Autodesk Inventor part; units mm, degrees
ref_plane "Start plane" through (0, 0, 0) normal (0, 0, 1) x (1, 0, 0)
ref_plane "End plane" through (0, 0, 900) normal (0, 0, 1) x (1, 0, 0)
ref_plane "YZ Plane" through (0, 0, 0) normal (1, 0, 0) x (0, 1, 0)
ref_plane "Start plane" through (0, 0, 0) normal (0, 0, 1) x (1, 0, 0)
ref_plane "End plane" through (0, 0, 900) normal (0, 0, 1) x (1, 0, 0)
sketch "Sketch" plane through (0, 0, 0) normal (0, 0, 1) x (1, 0, 0)
  line L0 (0.8698, -38.5) -> (-0.8698, -38.5)
  line L1 (2.2911, -16.445) -> (1.8696, -37.52)
  line L2 (13.04, -12.3892) -> (6.2103, -12.5258)
  line L3 (15, -8.5) -> (15, -10.3896)
  line L4 (-15, -10.3896) -> (-15, -8.5)
  line L5 (-6.2103, -12.5258) -> (-13.04, -12.3892)
  line L6 (-1.8696, -37.52) -> (-2.2911, -16.445)
  line L7 (-2.3679, -12.6026) -> (2.3679, -12.6026) construction
  line L8 (0, -46.445) -> (0, 7.7408) construction
  arc A0 (-2.2911, -16.445) -> (-6.2103, -12.5258) centre (-6.2903, -16.525) ccw
  arc A1 (6.2103, -12.5258) -> (2.2911, -16.445) centre (6.2903, -16.525) ccw
  arc A2 (-15, -10.3896) -> (-13.04, -12.3892) centre (-13, -10.3896) ccw
  arc A3 (13.04, -12.3892) -> (15, -10.3896) centre (13, -10.3896) ccw
  arc A4 (-1.8696, -37.52) -> (-0.8698, -38.5) centre (-0.8698, -37.5) ccw
  arc A5 (0.8698, -38.5) -> (1.8696, -37.52) centre (0.8698, -37.5) ccw
  line L9 (-21.5716, 0) -> (21.5716, 0) construction
  line L10 (-15, -8.5) -> (15, -8.5)
  point P0 (1.85, -38.5)
  point P1 (-1.85, -38.5)
  point P2 (15, -12.35)
  point P3 (-15, -12.35)
  point P4 (0, 0)
  point P5 (0, -12.6026)
  dimension "d9" = 3.85
  dimension "d11" = 3.85
  dimension "d23" = 3.7
  dimension "d26" = 1.146
  dimension "d27" = 1.146
  dimension "d28" = 4
  dimension "d29" = 2
  dimension "d30" = 1
  dimension "d31" = 30
  dimension "d32" = 1.146
  dimension "d33" = 30
  dimension "d34" = 8.5
extrude "Body" add sketch "Sketch" along normal up to surface (900 mm away) from surface at 0
sketch "Sketch3" plane through (0, 0, 0) normal (0, 0, 1) x (1, 0, 0)
  line L0 (0, 0) -> (10, 0)
ref_plane "Work Plane6" through (0, 0, 0) normal (0, -1, 0) x (1, 0, 0)
sketch "Sketch4" plane through (0, 0, 0) normal (0, -1, 0) x (1, 0, 0)
  line L0 (-2, 0) -> (12, 0)
  line L1 (-2, 900) -> (12, 900)
  dimension "d38" = 900
equation "\"d26\" = d27"
equation "\"d27\" = d32"
equation "\"d28\" = R"
equation "\"d29\" = R1"
equation "\"d30\" = R2"
equation "\"d32\" = msp_ang"
equation "\"d33\" = b"
equation "\"d34\" = ex"
equation "\"d13\" = G_L"
equation "\"b\" = 30"
equation "\"ParH\" = 30"
equation "\"R\" = 4"
equation "\"ParT\" = 4"
equation "\"R1\" = 2"
equation "\"R2\" = 1"
equation "\"G_L\" = d38"
equation "\"msp_x1\" = 0"
equation "\"msp_x2\" = 0"
equation "\"msp_x\" = 0"
equation "\"msp_ang\" = 1.14576deg"
equation "\"ex\" = 8.5"
equation "\"G_OFFSET_START\" = 0"
equation "\"G_OFFSET_END\" = 0"
properties part number "DIN 1024 - T30-900" material "Steel, Mild"
Model file for the job. Use its own axes, mm. Coordinates: 2 decimals unless noted, no trailing zeros. Loops run counter-clockwise (first coordinate to the right, second up) from the corner with the lowest first, then second, coordinate; pieces in that order, holes last. Notation, with made-up numbers: (26.5, 44) - (77.5, 44) arc R17 ccw to (77.5, 72) - close; hole circle Ø9 at (60, 43.25). An arc over 180 degrees is marked (long way). Write item = value, one per line. Start each with the question number.
Item 1: Saw through at A-A, the plane z = 225. List the corners of the cut face in (x, y) (3 decimals).
Item 2: Drop flat-ended pins along their axis: pin 1 Ø2 at (x, z) = (11, 616) entering from -Y; pin 2 Ø4 at (y, z) = (-25, 272.5) entering from +X; pin 3 Ø10 at (y, z) = (-22, 299.5) entering from -X. Give the stop position or say it passes through.
Item 3: Saw through at B-B, the plane y = -29. List the corners of the cut face in (x, z).
Item 4: Wall check: probe 1 along X at (y, z) = (-29.75, 293.5) (3 decimals); probe 2 along Y at (x, z) = (-10.25, 814) (3 decimals); probe 3 along X at (y, z) = (-22, 652.5). Give the ranges that are in metal, low to high. Write a range as [from, to].
Answers:
q1.outline = (-15, -10.39) arc R2 ccw to (-13.04, -12.389) - (-6.21, -12.526) arc R4 cw to (-2.291, -16.445) - (-1.87, -37.52) arc R1 ccw to (-0.87, -38.5) - (0.87, -38.5) arc R1 ccw to (1.87, -37.52) - (2.291, -16.445) arc R4 cw to (6.21, -12.526) - (13.04, -12.389) arc R2 ccw to (15, -10.39) - (15, -8.5) - (-15, -8.5) - close
q2.pin_1 = -12.45
q2.pin_2 = 2.16
q2.pin_3 = -2.28
q3.outline = (-2.04, 0) - (2.04, 0) - (2.04, 900) - (-2.04, 900) - close
q4.probe_1 = [-2.025, 2.025]
q4.probe_2 = [-12.445, -8.5]
q4.probe_3 = [-2.18, 2.18]
